The listing builds one solid part. Answer for the finished solid, in the listing's coordinates (mm). Face numbers are marked on the shaded views. A direction names the side the tool comes from. Round coordinates to 2 decimals unless told otherwise and drop trailing zeros. Order: outer loops, then holes, each group sorted by start corner. A loop starts at its lowest first (then second) coordinate and runs counter-clockwise, first axis right, second up. Notation, with made-up numbers: (31, 76) -> (86, 76) arc R18 ccw to (86, 84) -> close; hole circle Ø3 at (86, 46). An arc over 180 degrees is marked (long way). Return JSON: item names as keys, results as strings. Group by question number.
(1) The part is cut by section A-A (z = 19.25). Determine the outline of the cut face in (x, y).
(2) The part is cut by section C-C (z = 4.75). Count the separate pieces of the cut face and the enclosed holes in it, plus the area to 3 significant figures.
(3) Determine the mould class of the marked faces 1, 2 and 3 for opening direction X: +X half, -X half, draft (parallel to the pull), parting line (faces both ways), or undercut.
(4) The part is cut by section D-D (y = -16.5). Determine the outline of the cut face in (x, z), plus the area to 3 significant figures.
(5) Which of the six approach directions +Z, -Z, +X, -X, +Y, -Y give full straight-line access (tool end or side, diameter ignored) to the marked faces 4 and 5?
(6) Consider line 1 (Y direction, x = 0, z = 9.75); line 2 (X direction, y = 0, z = 16). Determine where each line is inside the solid, lowest interval first. Write a range as [from, to].
(7) Each of these flat-tipped pins is pushed along its axis until it touches: pin 1 (1 mm diameter, centred on x = -10, z = 9, fed in from -Y); pin 2 (8 mm diameter, centred on x = -3.5, z = 11, fed in from +Y); pin 3 (12 mm diameter, centred on y = 5.5, z = 13.5, fed in from -X). Where does it stop, or does it pass through?
(8) The part is cut by section B-B (y = 0). Determine the outline of the cut face in (x, z).
from build123d import *

# Parameters (mm, degrees)
F2_R     = 2.5
F3_DEPTH = 25


with BuildPart() as f1:
    # F0 (on Front) → F1 (revolve)
    with BuildSketch(Plane.XZ):
        Polygon((-20, 0), (-4.2, 0), (-4.2, 23.283258), (-8.2, 23.283258), (-14, 15), (-14, 4), (-20, 4), align=None)
    revolve(axis=Axis((0, 0, 31.447405), (0, 0, 1)))

    # F2 (on Top) → F3 (cut)
    with BuildSketch(Plane.XY):
        with Locations((0, -10)):
            Circle(F2_R)
        with Locations((7.071068, -7.071068)):
            Circle(F2_R)
        with Locations((10, 0)):
            Circle(F2_R)
        with Locations((7.071068, 7.071068)):
            Circle(F2_R)
        with Locations((0, 10)):
            Circle(F2_R)
        with Locations((-7.071068, 7.071068)):
            Circle(F2_R)
        with Locations((-10, 0)):
            Circle(F2_R)
        with Locations((-7.071068, -7.071068)):
            Circle(F2_R)
    extrude(amount=F3_DEPTH, mode=Mode.SUBTRACT)


solid = f1.part
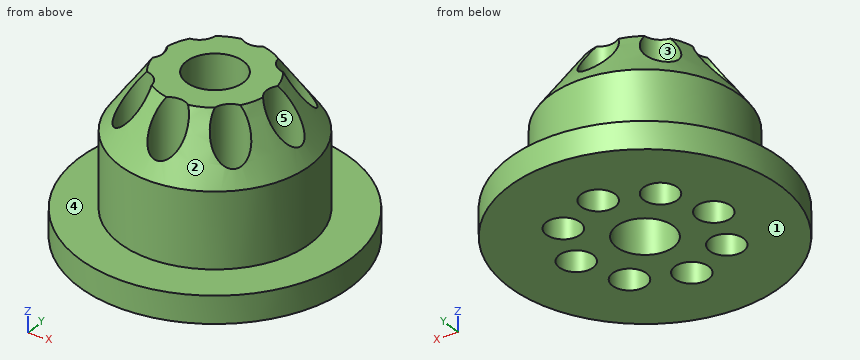
Answer below:
{
 "1": {"outline": "(-10.76, -2.38) arc R11.02 ccw to (-9.29, -5.93) arc R2.5 cw (long way) to (-5.93, -9.29) arc R11.02 ccw to (-2.38, -10.76) arc R2.5 cw (long way) to (2.38, -10.76) arc R11.02 ccw to (5.93, -9.29) arc R2.5 cw (long way) to (9.29, -5.93) arc R11.02 ccw to (10.76, -2.38) arc R2.5 cw (long way) to (10.76, 2.38) arc R11.02 ccw to (9.29, 5.93) arc R2.5 cw (long way) to (5.93, 9.29) arc R11.02 ccw to (2.38, 10.76) arc R2.5 cw (long way) to (-2.38, 10.76) arc R11.02 ccw to (-5.93, 9.29) arc R2.5 cw (long way) to (-9.29, 5.93) arc R11.02 ccw to (-10.76, 2.38) arc R2.5 cw (long way) to start; hole circle Ø8.4 at (0, 0)"},
 "2": {"separate pieces": "1", "enclosed holes": "9", "area": "403 mm²"},
 "3": {"face 1": "draft", "face 2": "parting line", "face 3": "undercut"},
 "4": {"outline": "(-11.3, 0) -> (11.3, 0) -> (11.3, 4) -> (-11.3, 4) -> close", "area": "90.4 mm²"},
 "5": {"face 4": "+Z", "face 5": "+Z, -Z"},
 "6": {"line 1": "y = [-14, -12.5], [-7.5, -4.2], [4.2, 7.5], [12.5, 14]", "line 2": "x = [-13.3, -12.5], [-7.5, -4.2], [4.2, 7.5], [12.5, 13.3]"},
 "7": {"pin 1": "stops at y = -10.28", "pin 2": "stops at y = 14", "pin 3": "stops at x = -14"},
 "8": {"outline": "(-20, 0) -> (-12.5, 0) -> (-12.5, 17.14) -> (-14, 15) -> (-14, 4) -> (-20, 4) -> close; (-7.5, 0) -> (-4.2, 0) -> (-4.2, 23.28) -> (-7.5, 23.28) -> close; (4.2, 0) -> (7.5, 0) -> (7.5, 23.28) -> (4.2, 23.28) -> close; (12.5, 0) -> (20, 0) -> (20, 4) -> (14, 4) -> (14, 15) -> (12.5, 17.14) -> close"}
}
